The listing builds one solid part. Answer for the finished solid, in the listing's coordinates (mm). Face numbers are marked on the shaded views. A direction names the side the tool comes from. Give positions to 0.01 mm unless a question says otherwise; leave off trailing zeros. Write each loop counter-clockwise with the first axis right and the second up, starting at its lowest first coordinate (ties: lowest second). Pieces come first, ordered by that corner, then holes. Notation, with made-up numbers: (88.5, 51) - (133.5, 51) arc R35 cw to (133.5, 84) - close; hole circle Ø4 at (6.5, 88.5). An arc over 180 degrees is marked (long way). One line per item, written item: value. Start each with the question number.
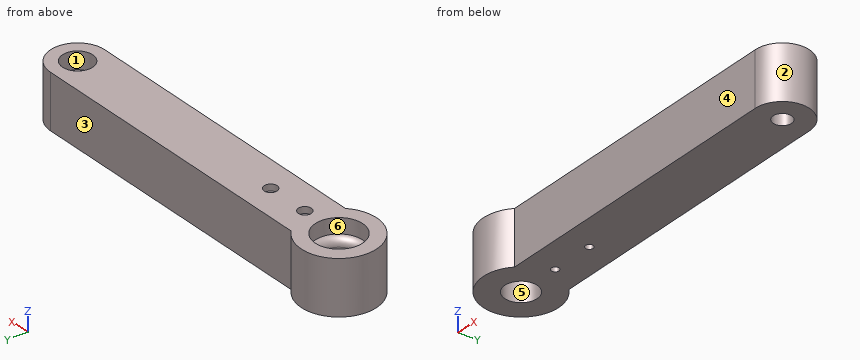
Autodesk Inventor part; units mm, degrees
ref_plane "YZ Plane" through (0, 0, 0) normal (1, 0, 0) x (0, 1, 0)
ref_plane "XZ Plane" through (0, 0, 0) normal (0, 1, 0) x (-1, 0, 0)
ref_plane "XY Plane" through (0, 0, 0) normal (0, 0, 1) x (1, 0, 0)
sketch "Sketch1" plane through (0, 0, 0) normal (0, 0, 1) x (1, 0, 0)
  line L0 (0, 12.6) -> (153, 12.6)
  arc A0 (153, -12.6) -> (153, 12.6) centre (153, 0) ccw
  line L1 (153, -12.6) -> (0, -12.6)
  arc A1 (0, 12.6) -> (0, -12.6) centre (0, 0) ccw
  circle A2 centre (0, 0) radius 7.5
  circle A3 centre (153, 0) radius 4.25
  dimension "d0" = 153
  dimension "d2" = 12.6
  dimension "d3" = 15
  dimension "d4" = 8.5
extrude "Extrusion1" add sketch "Sketch1" along normal blind 25
sketch "Sketch2" plane through (0, 0, 25) normal (0, 0, 1) x (1, 0, 0)
  circle A0 centre (0, 0) radius 7.5
  arc A1 (0, 12.6) -> (0, -12.6) centre (0, 0) ccw
  circle A2 centre (0, 0) radius 11
  dimension "d7" = 22
extrude "Extrusion2" cut sketch "Sketch2" against normal blind 7
sketch "Sketch4" plane through (0, 0, 25) normal (0, 0, 1) x (1, 0, 0)
  circle A0 centre (0, 0) radius 11
  circle A1 centre (20, 0) radius 1.75
  circle A2 centre (40, 0) radius 1.75
  dimension "d16" = 20
  dimension "d17" = 40
  dimension "d23" = 3.5
extrude "Extrusion3" cut sketch "Sketch4" against normal through all contours A1 | A2
sketch "Sketch5" plane through (0, 0, 25) normal (0, 0, 1) x (1, 0, 0)
  circle A0 centre (20, 0) radius 1.75
  circle A1 centre (40, 0) radius 1.75
  circle A2 centre (40, 0) radius 3
  circle A3 centre (20, 0) radius 3
  dimension "d28" = 6
extrude "Extrusion4" cut sketch "Sketch5" against normal blind 3
sketch "Sketch6" plane through (0, 0, 25) normal (0, 0, 1) x (1, 0, 0)
  line L0 (153, 12.6) -> (0, 12.6)
  arc A0 (0, 12.6) -> (0, -12.6) centre (0, 0) ccw
  line L1 (0, -12.6) -> (153, -12.6)
  arc A1 (12.1445, 12.6) -> (12.1445, -12.6) centre (0, 0) ccw
  dimension "d24" = 35
extrude "Extrusion5" add sketch "Sketch6" against normal up to surface (25 mm away)
sketch "Sketch7" plane through (0, 0, 25) normal (0, 0, 1) x (1, 0, 0)
  circle A0 centre (153, 0) radius 4.25
  arc A1 (153, -12.6) -> (153, 12.6) centre (153, 0) ccw
  circle A2 centre (153, 0) radius 7
  dimension "d30" = 14
extrude "Extrusion6" cut sketch "Sketch7" against normal blind 8
fillet "Fillet1" radius 3.5 1 edges at (-7.5, 0, 18)
properties part number "driven arm"
Item 1: Find section C-C on y = 0. Give the number of separate pieces and of enclosed holes in the cut face, plus the area to 3 significant figures.
Item 2: Find section B-B on z = 2.25. Determine the outline of the cut face in (x, y).
Item 3: For the marked faces 1 and 2, determine the directions among +Z, -Z, +X, -X, +Y, -Y from which every point of the face is accessible in a straight line to the end or side of a thin tool.
Item 4: The mould has two halves that part along Y. Classify the marked faces 3, 4, 5 and 6: +Y half, -Y half, draft (parallel to the pull), parting line (faces both ways), or undercut.
Item 5: Each of these flat-tipped pins is pushed along its axis until it touches: pin 1 Ø3 at (x, z) = (2, 3.5) entering from -Y; pin 2 Ø3 at (x, y) = (39.5, -1) entering from +Z; pin 3 Ø3 at (y, z) = (-2.5, 19.5) entering from +X; pin 4 Ø3 at (x, y) = (40, 0) entering from +Z. Where does it stop, or does it pass through?
Item 6: Find section A-A on x = 20. Determine the outline of the cut face in (y, z), plus the area to 3 significant figures.
Item 7: Straight lines are drawn through the part: line 1 along Y through (x, z) = (0, 23.5); line 2 along Y through (x, z) = (153, 3.5); line 3 along X through (y, z) = (3, 19.5). For each, find the intervals that lie inside material, in ascending order.
Values:
1. separate pieces: 5
1. enclosed holes: 0
1. area: 3,700 mm^2
2. outline: (12.14, -12.6) - (153, -12.6) arc R12.6 ccw to (153, 12.6) - (12.14, 12.6) arc R17.5 ccw (long way) to start; hole circle Ø15 at (0, 0); hole circle Ø3.5 at (20, 0); hole circle Ø3.5 at (40, 0); hole circle Ø8.5 at (153, 0)
3. face 1: +Z
3. face 2: +Z, -Z, +X
4. face 3: +Y half
4. face 4: -Y half
4. face 5: undercut
4. face 6: undercut
5. pin 1: y = -17.49
5. pin 2: z = 22
5. pin 3: x = 165.56
5. pin 4: through
6. outline: (-12.6, 0) - (-1.75, 0) - (-1.75, 22) - (-3, 22) - (-3, 25) - (-12.6, 25) - close; (1.75, 0) - (12.6, 0) - (12.6, 25) - (3, 25) - (3, 22) - (1.75, 22) - close
6. area: 535 mm^2
7. line 1: -17.5 to -11, 11 to 17.5
7. line 2: -12.6 to -4.25, 4.25 to 12.6
7. line 3: -17.24 to -10.58, 10.58 to 146.68, 159.32 to 165.24
